Job drawing, mm, ordinate dimensions from the low corner. One solid piece. A direction names the side the tool comes from. Round coordinates to 2 decimals unless told otherwise and drop trailing zeros. Order: outer loops, then holes, each group sorted by start corner. A loop starts at its lowest first (then second) coordinate and runs counter-clockwise, first axis right, second up. Notation, with made-up numbers: (42.5, 53) - (74.5, 53) arc R18 ccw to (74.5, 64) - close; hole circle Ø3 at (48, 19.5). An arc over 180 degrees is marked (long way). Write each question's results on one line, items separated by ' | '. Start each with the question number.
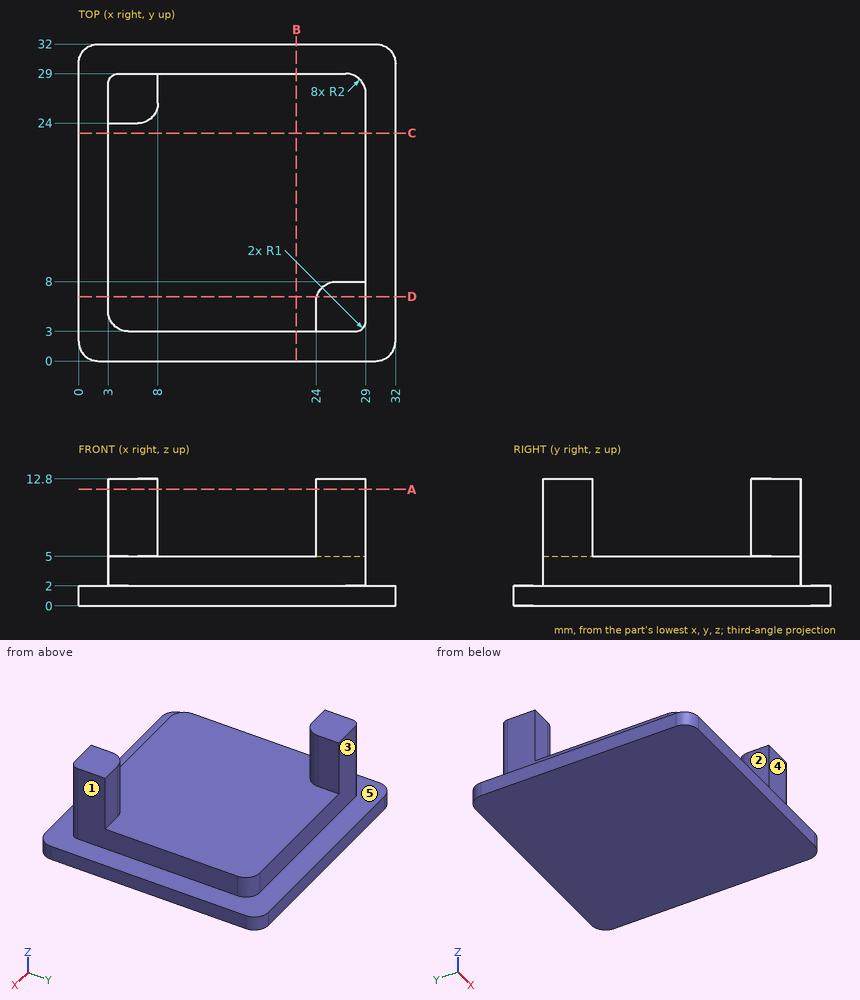
1. Cut at A-A (z = 11.75). List the corners of the cut face in (x, y).
2. Cut at D-D (y = 6.5). List the corners of the cut face in (x, z).
3. 3-axis set-ups, long thin cutter, end or side, ignore diameter. For the marked faces 1, 2, 3, 4 and 5: which of +Z, -Z, +X, -X, +Y, -Y reach the whole face in a straight line?
4. Cut at B-B (x = 22). List the corners of the cut face in (y, z).
5. Wall check: line 1 (Z direction, x = 26.5, y = 18.5); line 2 (X direction, y = 16, z = 2.25); line 3 (Z direction, x = 15, y = 1.5). Give the ranges that are in metal, low to high. Write a range as from..to.
6. Flat gauge pins, fed straight in: pin 1 Ø0.9 at (x, z) = (28, 10.5) entering from +Y; pin 2 Ø10 at (x, y) = (22, 8.5) entering from +Z; pin 3 Ø0.9 at (y, z) = (5, 10.5) entering from -X; pin 4 Ø0.9 at (x, z) = (4.5, 7) entering from -Y. Where does each tip first touch, or does it go through?
A:
1) outline: (3, 24) - (6, 24) arc R2 ccw to (8, 26) - (8, 29) - (4, 29) arc R1 ccw to (3, 28) - close; (24, 3) - (28, 3) arc R1 ccw to (29, 4) - (29, 8) - (26, 8) arc R2 ccw to (24, 6) - close
2) outline: (0, 0) - (32, 0) - (32, 2) - (29, 2) - (29, 12.8) - (24.06, 12.8) - (24.06, 5) - (3, 5) - (3, 2) - (0, 2) - close
3) face 1: +Z, +X, +Y, -Y | face 2: +Z, -X, +Y, -Y | face 3: +Z, +X, -X, +Y | face 4: +Z, +X, -X, -Y | face 5: +Z
4) outline: (0, 0) - (32, 0) - (32, 2) - (29, 2) - (29, 5) - (3, 5) - (3, 2) - (0, 2) - close
5) line 1: z = 0..5 | line 2: x = 3..29 | line 3: z = 0..2
6) pin 1: stops at y = 8 | pin 2: stops at z = 12.8 | pin 3: stops at x = 24 | pin 4: stops at y = 24
